Geometry check sheet. Reference: the model listing, model coordinates, mm. Round coordinates to 2 decimals unless told otherwise and drop trailing zeros. Order: outer loops, then holes, each group sorted by start corner. A loop starts at its lowest first (then second) coordinate and runs counter-clockwise, first axis right, second up. Notation, with made-up numbers: M -40,20.25 L -6,20.25 A25 cw -6,57.25 Z; hole C -32.5,-29.5 d6. An arc over 180 degrees is marked long. Return JSON: item names as keys, results as strings. Group by question number.
```python
from build123d import *

# Parameters (mm, degrees)
ESQUISSE1_R        = 9.5
BOSS_EXTRU_1_DEPTH = 30
CONG_1_R           = 1
ECHELLE1_SCALE     = 10


with BuildPart() as part:
    # Esquisse1 → Boss.-Extru.1 (new body)
    with BuildSketch(Plane(origin=(0, 0, 0), x_dir=(1, 0, 0), z_dir=(0, 1, 0))):
        Circle(ESQUISSE1_R)
    extrude(amount=BOSS_EXTRU_1_DEPTH)

    # Congé1
    cong_1_edges = [part.edges().sort_by_distance(p)[0] for p in [
        (-9.5, 0, 0),
    ]]
    fillet(cong_1_edges, radius=CONG_1_R)


with BuildPart() as part_1:
    # Echelle1: scaled about (0, 0, 0)
    add(part.part.scale(ECHELLE1_SCALE))


solid = part_1.part
```
Q1. Section check A-A on y = 273. Record the cut outline in (x, z).
Q2. Depth check by flat-ended pin: pin 1 Ø1.5 at (x, z) = (-2.5, -50.5) entering from -Y; pin 2 Ø5 at (x, y) = (12, 30) entering from +Z; pin 3 Ø1 at (y, z) = (246, 23) entering from -X; pin 4 Ø1 at (y, z) = (52, 22.5) entering from -X. Enter the tip coordinate at first touch or a pass-through.
Q3. Material ranges on line 1 along X through (y, z) = (19.5, 3); line 2 along X through (y, z) = (32.5, -69); line 3 along Z through (x, y) = (-60, 212), recorded low to high.
Geometry check:
{
 "1": {"outline": "C 0,0 d190"},
 "2": {"pin 1": "stops at y = 0", "pin 2": "stops at z = 94.52", "pin 3": "stops at x = -92.3", "pin 4": "stops at x = -92.42"},
 "3": {"line 1": "x = -94.95 to 94.95", "line 2": "x = -65.3 to 65.3", "line 3": "z = -73.65 to 73.65"}
}
